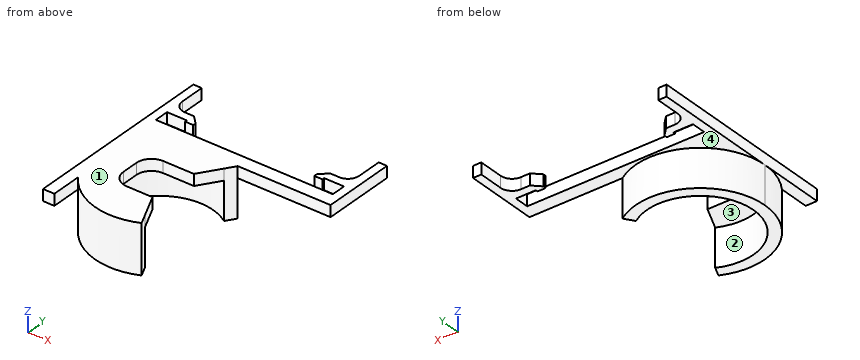
from build123d import *

# Parameters (mm, degrees)
F0_W     = 1.1
F0_H     = 4.7914452539
F1_DEPTH = 1.5
F2_SIZE  = 1
F3_R     = 1.5
F5_DEPTH = 1.5
F6_DEPTH = 5
F7_R     = 2


# Not quite as in the source:
# - a feature names something its author has since deleted; it is built from what else it names


with BuildPart() as f1:
    # F0 (on Top) → F1 (new body)
    with BuildSketch(Plane.XY):
        with BuildLine():
            ThreePointArc((-8.55, 0), (-4.0253321977, 7.5431558845), (4.7597545494, 7.1026218138))
            Line((4.7597545494, 7.1026218138), (4.7907789053, 7.1026218138))
            Line((4.7907789053, 7.1026218138), (6.0061305772, 8.9044547655))
            Line((6.0061305772, 8.9044547655), (-7.45, 8.9044547655))
            Line((-7.45, 8.9044547655), (-7.45, 10.8044547655))
            Line((-7.45, 10.8044547655), (-4.820069465, 10.8044547655))
            Line((-4.820069465, 10.8044547655), (-4.820069465, 10.5132658899))
            Line((-4.820069465, 10.5132658899), (-3.75, 10.5044547655))
            Line((-3.75, 10.5044547655), (-3.75, 10.8044547655))
            Line((-3.75, 10.8044547655), (-3.75, 11.9085547461))
            Line((-3.75, 11.9085547461), (-7.45, 11.9085547461))
            Line((-7.45, 11.9085547461), (-8.55, 11.9085547461))
            Line((-8.55, 11.9085547461), (-8.55, 10.5085547461))
            Line((-8.55, 10.5085547461), (-8.55, 0))
        make_face()
        with BuildLine():
            Line((-7.05, -8.869094649), (-7.05, -4.837354649))
            ThreePointArc((-7.05, -4.837354649), (-8.1663945533, -2.5322914524), (-8.55, 0))
            Line((-8.55, 0), (-8.55, -8.869094649))
            Line((-8.55, -8.869094649), (-7.05, -8.869094649))
        make_face()
        with BuildLine():
            ThreePointArc((2.9794587453, -6.3894698986), (-7.0282672028, 0.5531366249), (3.9423099695, 5.8447148865))
            Line((3.9423099695, 5.8447148865), (4.7810993247, 7.0882712453))
            ThreePointArc((4.7810993247, 7.0882712453), (4.7704323333, 7.0954545558), (4.7597545494, 7.1026218138))
            ThreePointArc((4.7597545494, 7.1026218138), (-4.0253321977, 7.5431558845), (-8.55, 0))
            ThreePointArc((-8.55, 0), (-8.1663945533, -2.5322914524), (-7.05, -4.837354649))
            ThreePointArc((-7.05, -4.837354649), (-2.2520876458, -8.248066515), (3.6133861379, -7.7489315792))
            Line((3.6133861379, -7.7489315792), (2.9794587453, -6.3894698986))
        make_face()
        Polygon((6.0061305772, 8.9044547655), (4.7907789053, 7.1026218138), (15.4494866027, 7.1026218138), (17.05, 7.1026218138), (17.05, 11.9085547461), (15.95, 11.9085547461), (12.25, 11.9085547461), (12.25, 10.8044547655), (12.25, 10.5044547655), (13.32, 10.5044547655), (13.32, 10.8044547655), (15.95, 10.8044547655), (15.95, 8.9044547655), align=None)
        with Locations((-8, 14.3042773731)):
            Rectangle(F0_W, F0_H)
        with Locations((16.5, 14.3042773731)):
            Rectangle(F0_W, F0_H)
    extrude(amount=F1_DEPTH)

    # F2
    f2_edges = [f1.edges().sort_by_distance(p)[0] for p in [
        (-3.75, 11.908555, 0.75),
        (12.25, 11.908555, 0.75),
    ]]
    chamfer(f2_edges, length=F2_SIZE)

    # F3
    f3_edges = [f1.edges().sort_by_distance(p)[0] for p in [
        (-7.45, 11.908555, 0.75),
        (15.95, 11.908555, 0.75),
    ]]
    fillet(f3_edges, radius=F3_R)

    # F4 (on face) → F5 (join)
    with BuildSketch(Plane.XY.offset(1.5)):
        with BuildLine():
            Line((2.0909764022, 3.1), (3.9423099695, 5.8447148865))
            ThreePointArc((3.9423099695, 5.8447148865), (-7.0282672028, 0.5531366249), (2.9794587453, -6.3894698986))
            Line((2.9794587453, -6.3894698986), (1.4455537403, -3.1))
            Line((1.4455537403, -3.1), (-3.96, -3.1))
            Line((-3.96, -3.1), (-3.96, 3.1))
            Line((-3.96, 3.1), (2.0909764022, 3.1))
        make_face()
    extrude(amount=-F5_DEPTH)

    # F0 (on Top) → F6 (join)
    with BuildSketch(Plane.XY):
        with BuildLine():
            ThreePointArc((2.9794587453, -6.3894698986), (-7.0282672028, 0.5531366249), (3.9423099695, 5.8447148865))
            Line((3.9423099695, 5.8447148865), (4.7810993247, 7.0882712453))
            ThreePointArc((4.7810993247, 7.0882712453), (4.7704323333, 7.0954545558), (4.7597545494, 7.1026218138))
            ThreePointArc((4.7597545494, 7.1026218138), (-4.0253321977, 7.5431558845), (-8.55, 0))
            ThreePointArc((-8.55, 0), (-8.1663945533, -2.5322914524), (-7.05, -4.837354649))
            ThreePointArc((-7.05, -4.837354649), (-2.2520876458, -8.248066515), (3.6133861379, -7.7489315792))
            Line((3.6133861379, -7.7489315792), (2.9794587453, -6.3894698986))
        make_face()
    extrude(amount=-F6_DEPTH)

    # F7
    f7_edges = [f1.edges().sort_by_distance(p)[0] for p in [
        (-3.96, 3.1, 0.75),
        (-3.96, -3.1, 0.75),
    ]]
    fillet(f7_edges, radius=F7_R)


solid = f1.part
Verification items for the finished model (mm, model axes). Face numbers are marked on the shaded views. A direction names the side the tool comes from. Coordinates: 2 decimals unless noted, no trailing zeros. Order: outer loops, then holes, each group sorted by start corner. A loop starts at its lowest first (then second) coordinate and runs counter-clockwise, first axis right, second up. Notation, with made-up numbers: M 33,65 L 87,65 A22 ccw 87,94 Z; hole C 0,4.5 d11. An arc over 180 degrees is marked long. One line per item, written item: value. Start each with the question number.
Item 1: Mould release check, pull along Y, two halves, no side actions. Record for the marked faces 3 and 4: pulls with the +Y half, pulls with the -Y half, needs draft (parallel to the pull), parting line crosses it, or undercut.
Item 2: Access from +Z, -Z, +X, -X, +Y, -Y to the whole of each face (thin tool, end or side, straight path). Record for the marked faces 1 and 2.
Item 3: Sectioned sample at A-A on x = 0. Record the cut outline in (y, z).
Item 4: Depth check by flat-ended pin: P1, Ø1.2, axis at x = 7.5, z = 0.5, coming from the +Y side; P2, Ø1.2, axis at x = 13, z = 1, coming from the -Y side; P3, Ø1, axis at x = -2, z = -2, coming from the -Y side; P4, Ø8, axis at x = 10.5, y = -6.5, coming from the -Z side. Enter the tip coordinate at first touch or a pass-through.
Item 5: Thickness scan on probe 1 along Y at (x, z) = (0, -2.55); probe 2 along X at (y, z) = (0, -1.95); probe 3 along Z at (x, y) = (-6.25, -1). Record the ranges inside material, lowest first.
Item 6: Sectioned sample at B-B on y = -5.75. Record the cut outline in (x, z).
Item 7: Sectioned sample at D-D on x = 6.25. Record the cut outline in (y, z), then the cut area to 3 significant figures.
Calculated:
1. face 3: undercut
1. face 4: needs draft
2. face 1: +Z, +X, -X, +Y, -Y
2. face 2: -Z
3. outline: M -8.55,-5 L -7.05,-5 L -7.05,0 L -3.1,0 L -3.1,1.5 L -8.55,1.5 Z; M 3.1,0 L 7.05,0 L 7.05,-5 L 8.55,-5 L 8.55,0 L 8.9,0 L 8.9,1.5 L 3.1,1.5 Z
4. P1: y = 8.9
4. P2: y = 7.1
4. P3: y = -8.42
4. P4: through
5. probe 1: -8.55 to -7.05, 7.05 to 8.55
5. probe 2: -8.55 to -7.05
5. probe 3: 0 to 1.5
6. outline: M -8.55,0 L -7.05,0 L -7.05,1.5 L -8.55,1.5 Z; M -6.33,-5 L -4.08,-5 L -4.08,0 L 2.68,0 L 2.68,1.5 L -6.33,1.5 Z
7. outline: M 7.1,0 L 8.9,0 L 8.9,1.5 L 7.1,1.5 Z
7. area: 2.70 mm^2
